Job drawing, mm, ordinate dimensions from the low corner. One solid piece. A direction names the side the tool comes from. Round coordinates to 2 decimals unless told otherwise and drop trailing zeros. Loops run counter-clockwise (first coordinate to the right, second up) from the corner with the lowest first, then second, coordinate; pieces in that order, holes last.
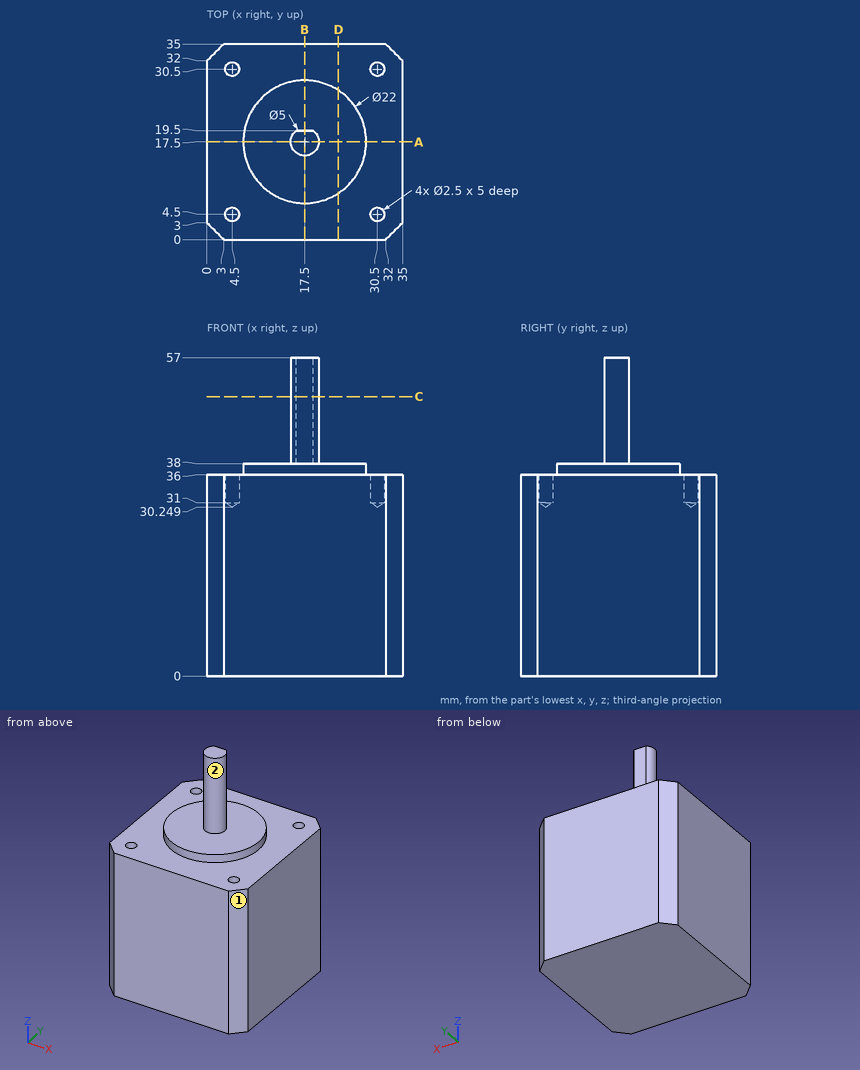
1) Slice it at A-A, the plane y = 17.5. Give the cut face in (x, z).
Values:
outline: (0, 0) - (35, 0) - (35, 36) - (28.5, 36) - (28.5, 38) - (20, 38) - (20, 57) - (15, 57) - (15, 38) - (6.5, 38) - (6.5, 36) - (0, 36) - close
2) Tool access for the marked faces 1 and 2: list every direction of +Z, -Z, +X, -X, +Y, -Y with a clear straight run to the whole face (end or side of a thin tool).
Values:
face 1: +Z, -Z, +X, -Y
face 2: +Z
3) Drop flat-ended pins along their axis: pin 1 Ø11 at (x, y) = (20.5, 22) entering from +Z; pin 2 Ø1 at (y, z) = (7.5, 39) entering from -X; pin 3 Ø10 at (y, z) = (19.5, 42) entering from +X; pin 4 Ø1.5 at (x, z) = (17, 47) entering from +Y. Give the stop position or say it passes through.
Values:
pin 1: stops at z = 57
pin 2: passes through
pin 3: stops at x = 28.5
pin 4: stops at y = 19.5
4) Slice it at C-C, the plane z = 50. Give the cut face in (x, y).
Values:
outline: (16, 19.5) arc R2.5 ccw (long way) to (19, 19.5) - close
5) Wall check: line 1 along X through (y, z) = (4.5, 34.5); line 2 along Z through (x, y) = (6, 8). Give the ranges that are in metal, low to high.
Values:
line 1: x = 0 to 3.25, 5.75 to 29.25, 31.75 to 35
line 2: z = 0 to 36
6) Slice it at D-D, the plane x = 23.5. Give the cut face in (y, z).
Values:
outline: (0, 0) - (35, 0) - (35, 36) - (26.72, 36) - (26.72, 38) - (8.28, 38) - (8.28, 36) - (0, 36) - close
7) Slice it at B-B, the plane x = 17.5. Give the cut face in (y, z), then the cut area to 3 significant figures.
Values:
outline: (0, 0) - (35, 0) - (35, 36) - (28.5, 36) - (28.5, 38) - (19.5, 38) - (19.5, 57) - (15, 57) - (15, 38) - (6.5, 38) - (6.5, 36) - (0, 36) - close
area: 1,390 mm2
